The listing builds one solid part. Answer for the finished solid, in the listing's coordinates (mm). Coordinates: 2 decimals unless noted, no trailing zeros. Order: outer loops, then holes, each group sorted by start corner. A loop starts at its lowest first (then second) coordinate and runs counter-clockwise, first axis right, second up. Notation, with made-up numbers: (18, 7) -> (60, 7) arc R31 cw to (60, 38) -> close; hole circle Ø6 at (2.25, -31). An arc over 180 degrees is marked (long way). Write item = value, one per line.
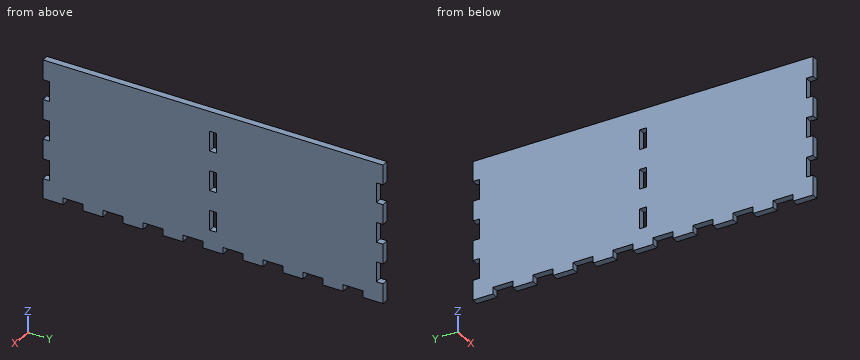
from build123d import *

# Parameters (mm, degrees)
F0_W     = 161.925
F0_H     = 66.675
F1_DEPTH = 3.175
F2_W     = 3.175
F2_H     = 9.525
F3_DEPTH = 3.176
F4_W     = 9.525
F4_H     = 3.175
F5_DEPTH = 3.176


with BuildPart() as f1:
    # F0 (on Right) → F1 (new body)
    with BuildSketch(Plane.YZ):
        Rectangle(F0_W, F0_H)
    extrude(amount=F1_DEPTH)

    # F2 (on face) → F3 (cut, through all)
    with BuildSketch(Plane.YZ.offset(3.175)):
        with Locations((-79.375, -19.05)):
            Rectangle(F2_W, F2_H)
        with Locations((-79.375, 0)):
            Rectangle(F2_W, F2_H)
        with Locations((-79.375, 19.05)):
            Rectangle(F2_W, F2_H)
        with Locations((0, -19.05)):
            Rectangle(F2_W, F2_H)
        Rectangle(F2_W, F2_H)
        with Locations((0, 19.05)):
            Rectangle(F2_W, F2_H)
        with Locations((79.375, -19.05)):
            Rectangle(F2_W, F2_H)
        with Locations((79.375, 0)):
            Rectangle(F2_W, F2_H)
        with Locations((79.375, 19.05)):
            Rectangle(F2_W, F2_H)
    extrude(amount=-F3_DEPTH, mode=Mode.SUBTRACT)

    # F4 (on face) → F5 (cut, through all)
    with BuildSketch(Plane.YZ.offset(3.175)):
        with Locations((-66.675, -31.75)):
            Rectangle(F4_W, F4_H)
        with Locations((-47.625, -31.75)):
            Rectangle(F4_W, F4_H)
        with Locations((-28.575, -31.75)):
            Rectangle(F4_W, F4_H)
        with Locations((-9.525, -31.75)):
            Rectangle(F4_W, F4_H)
        with Locations((9.525, -31.75)):
            Rectangle(F4_W, F4_H)
        with Locations((28.575, -31.75)):
            Rectangle(F4_W, F4_H)
        with Locations((47.625, -31.75)):
            Rectangle(F4_W, F4_H)
        with Locations((66.675, -31.75)):
            Rectangle(F4_W, F4_H)
    extrude(amount=-F5_DEPTH, mode=Mode.SUBTRACT)


solid = f1.part
Q1. Section A-A, the plane z = -20 is taken. Give the vertices of the cut face in (x, y) (1 decimal).
The answers:
outline = (0, -77.8) -> (3.2, -77.8) -> (3.2, -1.6) -> (0, -1.6) -> close; (0, 1.6) -> (3.2, 1.6) -> (3.2, 77.8) -> (0, 77.8) -> close
Q2. Each of these flat-tipped pins is pushed along its axis until it touches: pin 1 Ø1 at (x, z) = (2, -20) entering from +Y; pin 2 Ø1 at (x, y) = (1.5, -49) entering from -Z. Where does it stop, or does it pass through?
The answers:
pin_1 = 77.79
pin_2 = -30.16
Q3. Section B-B, the plane y = 50 is taken. Give the vertices of the cut face in (x, z) (1 decimal), plus the area to 3 significant figures.
The answers:
outline = (0, -30.2) -> (3.2, -30.2) -> (3.2, 33.3) -> (0, 33.3) -> close
area = 202 mm2
Q4. Find the intervals of material crossed by line 1 along Y through (x, z) = (2.9, 0.5); line 2 along Z through (x, y) = (0.8, -44.5), in increasing order.
The answers:
line_1 = -77.79 to -1.59, 1.59 to 77.79
line_2 = -30.16 to 33.34
Q5. Section C-C, the plane x = 2.55 is taken. Give the number of separate pieces and of enclosed holes in the cut face, plus the area to 3 significant figures.
The answers:
separate_pieces = 1
enclosed_holes = 3
area = 10,300 mm2
